Autodesk Inventor part; units mm, degrees
ref_plane "Work Plane1" through (0, -6.35, 57.7672) normal (0, 0, -1) x (0, 1, 0)
ref_plane "Work Plane2" through (2.413, 0, 64.1172) normal (0, 0, -1) x (-1, 0, 0)
ref_plane "YZ Plane" through (0, 0, 0) normal (1, 0, 0) x (0, 1, 0)
sketch "Sketch1" plane through (0, 0, 0) normal (0, 0, 1) x (1, 0, 0)
  arc A0 (-8.0491, 3.1697) -> (-8.0491, -3.1803) centre (-17.5665, -0.0053) ccw
  line L0 (-1.651, -3.1803) -> (-8.0491, -3.1803)
  line L1 (-1.651, -5.461) -> (-1.651, -3.1803)
  line L2 (0, -5.461) -> (-1.651, -5.461)
  line L3 (0, -5.461) -> (0, -6.35)
  line L4 (3.175, -6.35) -> (0, -6.35)
  line L5 (3.175, 6.35) -> (3.175, -6.35)
  line L6 (3.175, 6.35) -> (0, 6.35)
  line L7 (0, 6.35) -> (0, 5.461)
  line L8 (-1.651, 5.461) -> (0, 5.461)
  line L9 (-1.651, 3.1697) -> (-1.651, 5.461)
  line L10 (-1.651, 3.1697) -> (-8.0491, 3.1697)
  line L11 (3.175, 5.842) -> (0.508, 5.842)
  line L12 (0.508, 5.842) -> (0.508, -5.842)
  line L13 (0.508, -5.842) -> (3.175, -5.842)
  line L14 (3.175, -5.842) -> (3.175, 5.842)
  line L15 (0.508, 5.207) -> (1.651, 5.207)
  line L16 (1.651, 5.207) -> (1.651, -5.207)
  line L17 (1.651, -5.207) -> (0.508, -5.207)
  line L18 (0.508, -5.207) -> (0.508, 5.207)
  point P0 (0, 0)
  dimension "d0" = 0.508
  dimension "d1" = 0.508
  dimension "d2" = 0.508
  dimension "d3" = 0.635
  dimension "d4" = 0.635
  dimension "d5" = 1.524
ref_plane "Work Plane1" through (0, -6.35, 57.7672) normal (0, 0, -1) x (0, 1, 0)
extrude "Extrusion1" add sketch "Sketch1" along normal up to surface (57.7672 mm away) contours L5 L13 L12 L17 L16 L15 L11
ref_plane "Work Plane2" through (2.413, 0, 64.1172) normal (0, 0, -1) x (-1, 0, 0)
sketch "Sketch2" plane through (2.413, 0, 64.1172) normal (0, 0, -1) x (-1, 0, 0)
  line L0 (-0.762, -5.842) -> (-0.762, 5.842)
  line L1 (-0.762, 5.08) -> (3.556, 5.08)
  line L2 (3.556, 5.08) -> (3.556, 4.572)
  line L3 (3.556, 4.572) -> (-0.762, 4.572)
  line L4 (-0.762, 4.572) -> (-0.762, 5.08)
  line L5 (-0.762, -5.08) -> (3.556, -5.08)
  line L6 (3.556, -5.08) -> (3.556, -4.572)
  line L7 (3.556, -4.572) -> (-0.762, -4.572)
  line L8 (-0.762, -4.572) -> (-0.762, -5.08)
  line L9 (1.905, -5.207) -> (0.762, -5.207)
  line L10 (0.762, 5.207) -> (1.905, 5.207)
  line L11 (-0.762, 5.08) -> (0.508, 5.08)
  line L12 (0.508, 5.08) -> (0.508, -5.08)
  line L13 (0.508, -5.08) -> (-0.762, -5.08)
  line L14 (-0.762, -5.08) -> (-0.762, 5.08)
  point P0 (2.413, 0)
  dimension "d8" = 0.508
  dimension "d9" = 4.318
  dimension "d10" = 4.318
  dimension "d11" = 0.508
  dimension "d12" = 0.127
  dimension "d13" = 0.127
extrude "Extrusion2" add sketch "Sketch2" along normal up to surface (6.35 mm away)
sketch "Sketch3" plane through (1.651, -5.207, 0) normal (-1, 0, 0) x (0, 0, 1)
  line L0 (0, 10.414) -> (57.7672, 10.414)
  line L1 (57.7672, 10.414) -> (56.4972, 10.414)
  line L2 (56.4972, 10.414) -> (56.4972, 9.779)
  line L3 (56.4972, 9.779) -> (57.7672, 9.779)
  line L4 (57.7672, 9.779) -> (57.7672, 10.414)
  line L5 (57.7672, -0.635) -> (57.7672, 0.127)
  line L6 (57.7672, 0) -> (56.4972, 0)
  line L7 (56.4972, 0.635) -> (57.7672, 0.635)
  line L8 (57.7672, 0.635) -> (57.7672, 0)
  line L9 (64.1172, 9.779) -> (57.7672, 9.779)
  line L10 (56.4972, 0.635) -> (56.4972, 0)
  point P0 (0, 5.207)
  dimension "d16" = 1.27
extrude "Extrusion3" add sketch "Sketch3" along normal up to surface (1.143 mm away)
sketch "Sketch4" plane through (3.175, -5.842, 0) normal (1, 0, 0) x (0, 0, -1)
  line L0 (0, 11.684) -> (-57.7672, 11.684)
  line L1 (0.0018, 0) -> (-0.5062, 0)
  line L2 (-0.5062, 0) -> (-0.5062, 11.684)
  line L3 (-0.5062, 11.684) -> (0.0018, 11.684)
  line L4 (0.0018, 11.684) -> (0.0018, 0)
  point P0 (0, 5.842)
  dimension "d19" = 0.508
extrude "Extrusion4" cut sketch "Sketch4" against normal blind 25.4
sketch "Sketch5" plane through (3.175, -5.08, 64.1172) normal (1, 0, 0) x (0, 0, -1)
  line L0 (63.611, -0.762) -> (63.611, 10.922)
  line L1 (63.611, 10.922) -> (6.35, 10.922)
  line L2 (6.35, 10.16) -> (6.35, 10.922)
  line L3 (0, 10.16) -> (6.35, 10.16)
  line L4 (0, 10.16) -> (0, 0)
  line L5 (0, 0) -> (6.35, 0)
  line L6 (6.35, -0.762) -> (6.35, 0)
  line L7 (63.611, -0.762) -> (6.35, -0.762)
  line L8 (6.35, 10.16) -> (6.35, 10.922)
  line L9 (0, 9.652) -> (0, 10.16)
  line L10 (6.35, 10.922) -> (0, 10.922)
  line L11 (0, 10.922) -> (0, 10.16)
  line L12 (0, 10.16) -> (6.35, 10.16)
  line L13 (6.35, 10.16) -> (6.35, 10.922)
  line L14 (0, 10.16) -> (0, 0)
  line L15 (6.35, -0.762) -> (6.35, 0)
  line L16 (0, 0) -> (6.35, 0)
  line L17 (6.35, 0) -> (6.35, -0.762)
  line L18 (6.35, -0.762) -> (0, -0.762)
  line L19 (0, -0.762) -> (0, 0)
  point P0 (64.1172, 5.08)
extrude "Extrusion5" add sketch "Sketch5" against normal up to surface (4.318 mm away) contours L18 L19 L5 L6 | L2 L3 L11 L10
sketch "Sketch6" plane through (2.413, 0, 64.1172) normal (0, 0, 1) x (1, 0, 0)
  line L0 (-0.508, -4.572) -> (-0.508, 4.572)
  line L1 (-3.556, -4.572) -> (-0.508, -4.572)
  line L2 (-3.556, -4.572) -> (-3.556, -5.842)
  line L3 (0.762, -5.842) -> (-3.556, -5.842)
  line L4 (0.762, 5.842) -> (0.762, -5.842)
  line L5 (0.762, 5.842) -> (-3.556, 5.842)
  line L6 (-3.556, 4.572) -> (-3.556, 5.842)
  line L7 (-0.508, 4.572) -> (-3.556, 4.572)
  line L8 (0.762, -5.842) -> (-3.556, -5.842)
  line L9 (-3.556, -5.842) -> (-1.905, -5.842)
  line L10 (-1.905, -5.842) -> (-1.905, -5.207)
  line L11 (-1.905, -5.207) -> (-3.556, -5.207)
  line L12 (-3.556, -5.207) -> (-3.556, -5.842)
  line L13 (-3.556, 5.842) -> (-1.905, 5.842)
  line L14 (-1.905, 5.842) -> (-1.905, 5.207)
  line L15 (-1.905, 5.207) -> (-3.556, 5.207)
  line L16 (-3.556, 5.207) -> (-3.556, 5.842)
  line L17 (-1.905, 5.842) -> (-1.905, 5.207)
  line L18 (-1.905, 4.572) -> (-1.905, 5.207)
  line L19 (-1.905, 5.842) -> (-1.905, 4.572)
  line L20 (-1.905, -5.207) -> (-1.905, -5.842)
  line L21 (-1.905, -4.572) -> (-1.905, -5.842)
  line L22 (-1.905, -5.207) -> (-1.905, -4.572)
  line L23 (-0.762, -5.207) -> (-1.905, -5.207)
  line L24 (-1.905, -5.207) -> (-0.762, -5.207)
  line L25 (-1.905, 5.207) -> (-0.762, 5.207)
  line L26 (-0.762, 5.207) -> (-1.905, 5.207)
  point P0 (-2.413, 0)
extrude "Extrusion6" cut sketch "Sketch6" against normal blind 25.4 contours L10 L3 L2 L11 | L15 L6 L5 L14
properties part number "Wire Cover Strengthened"
Could you check a few things on this model? Use its own coordinates, in mm. A direction names the side the tool comes from. Round coordinates to 2 decimals unless told otherwise and drop trailing zeros. Loops run counter-clockwise (first coordinate to the right, second up) from the corner with the lowest first, then second, coordinate; pieces in that order, holes last.
Q1. On a 3-axis mill with a long thin cutter (end or side, diameter ignored), from which of +Z, -Z, +X, -X, +Y, -Y can I reach the whole of each face in a straight line? I mean faces 5 (the flat face through (1, -5.207, 28)), 6 (the flat face through (2, 5.842, 32)), 7 (the flat face through (0, 5.207, 61)). Say none if no direction works.
Q2. I want a section at D-D (z = 59). Write out the boundary of the cut face in (x, y) (3 decimals), and give its area (3 significant figures).
Q3. I want a section at C-C (z = 24). Write out the boundary of the cut face in (x, y) (3 decimals), and give its area (3 significant figures).
Q4. I want a section at B-B (y = 2.5). Write out the boundary of the cut face in (x, z) (3 decimals).
Q5. I want a section at A-A (x = -0.55). Write out the boundary of the cut face in (y, z), and give its area (3 significant figures).
Q6. Thinking about a two-plate mould opening in Y: for faces 1 (the flat face through (1.905, 0, 61)), 2 (the flat face through (1.651, 0, 29)), 3 (the flat face through (0, -5.207, 61)), 4 (the flat face through (2, 0, 0.506)), which applies, pulls with the +Y half, pulls with the -Y half, needs draft (parallel to the pull), parting line crosses it, or undercut?
Q7. For P1, Ø5, axis at y = 1.5, z = 61.5, coming from the -X side (3 decimals); P2, Ø0.8, axis at x = -0.5, z = 61.5, coming from the -Y side; P3, Ø0.6, axis at y = 5, z = 39.5, coming from the -X side, each with a flat end and sliding along its axis, tell me the tip position at first contact or that it passes through.
Q8. Please list where these lines run through material, in increasing order: L1, parallel to Y at x = -0.65, z = 59; L2, parallel to Y at x = 1.1, z = 17; L3, parallel to X at y = -3.5, z = 33 (3 decimals).
Answer below:
1. face 5: -Z, -X
1. face 6: +Z, -Z, +X, -X, +Y
1. face 7: +Z, -Z, -X, +Y
2. outline: (-1.143, -5.207) - (0.508, -5.207) - (0.508, -5.842) - (3.175, -5.842) - (3.175, 5.842) - (0.508, 5.842) - (0.508, 5.207) - (-1.143, 5.207) - (-1.143, 4.572) - (1.905, 4.572) - (1.905, -4.572) - (-1.143, -4.572) - close
2. area: 20.5 mm2
3. outline: (0.508, -5.842) - (3.175, -5.842) - (3.175, 5.842) - (0.508, 5.842) - (0.508, 5.207) - (1.651, 5.207) - (1.651, -5.207) - (0.508, -5.207) - close
3. area: 19.3 mm2
4. outline: (1.651, 0.506) - (3.175, 0.506) - (3.175, 64.117) - (1.905, 64.117) - (1.905, 57.767) - (1.651, 57.767) - close
5. outline: (-5.21, 57.77) - (-4.57, 57.77) - (-4.57, 64.12) - (-5.21, 64.12) - close; (4.57, 57.77) - (5.21, 57.77) - (5.21, 64.12) - (4.57, 64.12) - close
5. area: 8.06 mm2
6. face 1: undercut
6. face 2: undercut
6. face 3: pulls with the -Y half
6. face 4: needs draft
7. P1: stops at x = 1.905
7. P2: stops at y = -5.21
7. P3: stops at x = 0.51
8. L1: y = -5.21 to -4.57, 4.57 to 5.21
8. L2: y = -5.84 to -5.21, 5.21 to 5.84
8. L3: x = 1.651 to 3.175
